Verification items for this drawing (mm, ordinates from the low corner). Give positions to 0.01 mm unless a question says otherwise; leave off trailing zeros. Order: outer loops, then holes, each group sorted by start corner. A loop starts at its lowest first (then second) coordinate and runs counter-clockwise, first axis right, second up. Notation, with made-up numbers: (33, 33) - (40, 33) arc R26 ccw to (40, 63) - close; hole circle Ø4 at (6.5, 22). An arc over 180 degrees is marked (long way). Put each result on its own line as item: value. Start each with the question number.
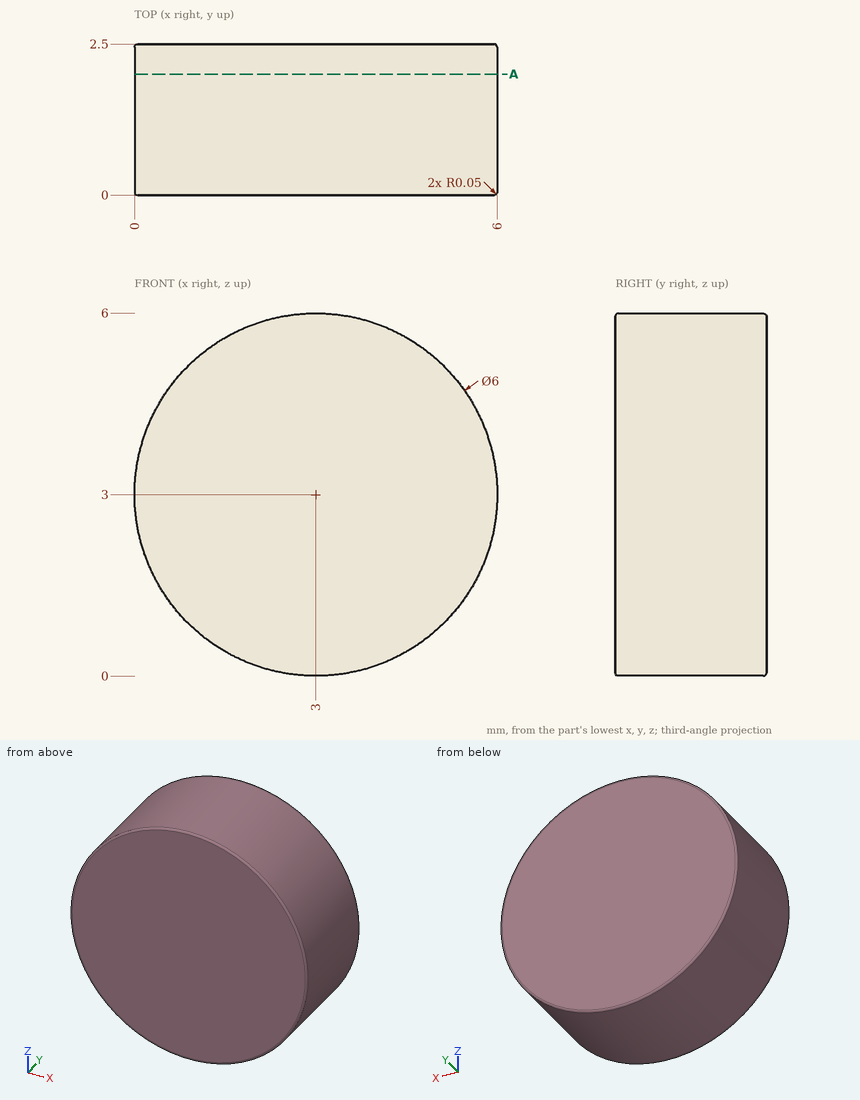
Item 1: Thickness scan on line 1 along X through (y, z) = (2.3, 4); line 2 along Z through (x, y) = (5, 1.5); line 3 along X through (y, z) = (2.15, 3.5). Record the ranges inside material, lowest first.
Item 2: Cross-section at A-A (y = 2). Enter the section's corners in (x, z).
Item 3: Gauge pin test, flat end, axial feed: pin 1 Ø1 at (y, z) = (1.5, 4) entering from -X. Record the tip position at first contact, or that the pin passes through.
Recorded:
1. line 1: x = 0.17 to 5.83
1. line 2: z = 0.76 to 5.24
1. line 3: x = 0.04 to 5.96
2. outline: circle Ø6 at (3, 3)
3. pin 1: stops at x = 0.04
